from build123d import *

# Parameters (mm, degrees)
BASE_FLANGE1_DEPTH         = 3.175
CUT_EXTRUDE1_DEPTH         = 194.329458355
CUT_EXTRUDE2_DEPTH         = 194.329458355
F_5_2_5_2_DIAMETER_HOLE1_D = 5.2
F_5_5_5_5_DIAMETER_HOLE1_D = 5.5


# Sheet-metal steps are written as plain solids
with BuildPart() as part:
    # Sketch11 → Base-Flange1 (new body)
    with BuildSketch(Plane.XZ.offset(-32.134736729)):
        with BuildLine():
            Line((-82.671285527, -32.35), (-104.922239506, -36.273443533))
            Line((-104.922239506, -36.273443533), (-104.922239506, -162.35))
            Line((-104.922239506, -162.35), (-24.333100178, -162.35))
            ThreePointArc((-24.333100178, -162.35), (-17.262032366, -159.421067812), (-14.333100178, -152.35))
            Line((-14.333100178, -152.35), (-14.333100178, -32.35))
            Line((-14.333100178, -32.35), (-82.671285527, -32.35))
        make_face()
    extrude(amount=-BASE_FLANGE1_DEPTH)

    # Sketch16 → Cut-Extrude1 (cut, through all)
    with BuildSketch(Plane(origin=(0, 35.309736729, 0), x_dir=(-1, 0, 0), z_dir=(0, 1, 0))):
        with BuildLine():
            Line((104.922239506, -142.35), (104.922239506, -56.273443533))
            Line((104.922239506, -56.273443533), (94.922239506, -56.273443533))
            ThreePointArc((94.922239506, -56.273443533), (87.851171694, -59.202375721), (84.922239506, -66.273443533))
            Line((84.922239506, -66.273443533), (84.922239506, -132.35))
            ThreePointArc((84.922239506, -132.35), (87.851171694, -139.421067812), (94.922239506, -142.35))
            Line((94.922239506, -142.35), (104.922239506, -142.35))
        make_face()
    extrude(amount=-CUT_EXTRUDE1_DEPTH, mode=Mode.SUBTRACT)

    # Sketch17 → Cut-Extrude2 (cut, through all)
    with BuildSketch(Plane(origin=(0, 35.309736729, 0), x_dir=(-1, 0, 0), z_dir=(0, 1, 0))):
        with BuildLine():
            Line((64.333100178, -128.85), (64.333100178, -68.85))
            ThreePointArc((64.333100178, -68.85), (49.333100178, -53.85), (34.333100178, -68.85))
            Line((34.333100178, -68.85), (34.333100178, -128.85))
            ThreePointArc((34.333100178, -128.85), (49.333100178, -143.85), (64.333100178, -128.85))
        make_face()
    extrude(amount=-CUT_EXTRUDE2_DEPTH, mode=Mode.SUBTRACT)

    # Ø5.2 (5.2) Diameter Hole1 (through all)
    with Locations(Plane(origin=(0, 32.134736729, 0), x_dir=(-1, 0, 0), z_dir=(0, -1, 0))):
        with Locations((94.922239506, 152.35), (74.922239506, 152.35)):
            Hole(F_5_2_5_2_DIAMETER_HOLE1_D / 2)

    # Ø5.5 (5.5) Diameter Hole1 (through all)
    with Locations(Plane(origin=(0, 32.134736729, 0), x_dir=(-1, 0, 0), z_dir=(0, -1, 0))):
        with Locations((95.316058397, 46.273443533), (74.375466886, 47.35), (24.333100178, 47.35), (24.333100178, 152.35)):
            Hole(F_5_5_5_5_DIAMETER_HOLE1_D / 2)


solid = part.part
Check sheet for the modelled part. Datum: model origin and axes. Units: mm. A direction names the side the tool comes from. Give positions to 0.01 mm unless a question says otherwise; leave off trailing zeros. Write each loop counter-clockwise with the first axis right and the second up, starting at its lowest first coordinate (ties: lowest second). Pieces come first, ordered by that corner, then holes. Notation, with made-up numbers: (-8, 4.25) -> (1, 4.25) arc R31 ccw to (1, 41.25) -> close; hole circle Ø2 at (1.25, 34.25). An arc over 180 degrees is marked (long way). Use one line per item in the form item = value. Start each with the question number.
1. Access from +Z, -Z, +X, -X, +Y, -Y to the whole of each face (thin tool, end or side, straight path). Record for faces 5 (the flat face through (-34.333, 34, -98)), 6 (the flat face through (-100, 34, -142.35)), 7 (the flat face through (-70, 35.31, -96)).
2. Thickness scan on line 1 along X through (y, z) = (32.95, -152.35); line 2 along X through (y, z) = (33.85, -76); line 3 along X through (y, z) = (34, -49.5). Record the ranges inside material, lowest first. Write a range as from..to.
3. Mould release check, pull along X, two halves, no side actions. Record for faces 1 (the cylindrical face through (-49.003, 33.744, -143.846)), 2 (the flat face through (-104.922, 34, -152)), 3 (the cylindrical face through (-17.34, 33.7, -159.5)), 4 (the cylindrical face through (-93.52, 33.74, -154.54)): pulls with the +X half, pulls with the -X half, needs draft (parallel to the pull), parting line crosses it, or undercut.
4. Section check C-C (y = 33.8). Record the cut outline in (x, z).
5. Section check A-A (z = -125.5). Record the cut outline in (x, y), and give its area (3 significant figures).
6. Go/stop test with flat-tipped pins: P1, Ø4.5, axis at x = -94.92, z = -152.35, coming from the +Y side; P2, Ø1.6, axis at y = 33, z = -92.5, coming from the -X side. Record where each tip stops, or that it passes through.
7. Section check B-B (x = -51). Record the cut outline in (y, z).
Conclusion:
q1.face_5 = +Y, -Y
q1.face_6 = -X, +Y, -Y
q1.face_7 = +Z, -Z, +X, -X, +Y
q2.line_1 = -104.92..-97.52, -92.32..-77.52, -72.32..-27.08, -21.58..-14.33
q2.line_2 = -84.92..-64.33, -34.33..-14.33
q2.line_3 = -104.92..-76.09, -72.66..-26.05, -22.62..-14.33
q3.face_1 = undercut
q3.face_2 = pulls with the -X half
q3.face_3 = pulls with the +X half
q3.face_4 = undercut
q4.outline = (-104.92, -162.35) -> (-24.33, -162.35) arc R10 ccw to (-14.33, -152.35) -> (-14.33, -32.35) -> (-82.67, -32.35) -> (-104.92, -36.27) -> (-104.92, -56.27) -> (-94.92, -56.27) arc R10 cw to (-84.92, -66.27) -> (-84.92, -132.35) arc R10 cw to (-94.92, -142.35) -> (-104.92, -142.35) -> close; hole circle Ø5.5 at (-95.32, -46.27); hole circle Ø5.2 at (-94.92, -152.35); hole circle Ø5.2 at (-74.92, -152.35); hole circle Ø5.5 at (-74.38, -47.35); hole (-64.33, -128.85) arc R15 ccw to (-34.33, -128.85) -> (-34.33, -68.85) arc R15 ccw to (-64.33, -68.85) -> close; hole circle Ø5.5 at (-24.33, -152.35); hole circle Ø5.5 at (-24.33, -47.35)
q5.outline = (-84.92, 32.13) -> (-64.33, 32.13) -> (-64.33, 35.31) -> (-84.92, 35.31) -> close; (-34.33, 32.13) -> (-14.33, 32.13) -> (-14.33, 35.31) -> (-34.33, 35.31) -> close
q5.area = 129 mm²
q6.P1 = through
q6.P2 = -84.92
q7.outline = (32.13, -162.35) -> (35.31, -162.35) -> (35.31, -143.76) -> (32.13, -143.76) -> close; (32.13, -53.94) -> (35.31, -53.94) -> (35.31, -32.35) -> (32.13, -32.35) -> close
